Model file for the job. Use its own axes, mm. A direction names the side the tool comes from. Give positions to 0.01 mm unless a question says otherwise; leave off trailing zeros. One line per item, written item: value. Start each with the question number.
(1) Probe L1, parallel to Z at x = 12.5, y = -4.75; L2, parallel to Z at x = 19, y = -5.25; L3, parallel to X at y = -4.25, z = 24. List the from-to ranges inside material, lowest first.
(2) Cut at A-A, the plane x = -9. State how many separate pieces and enclosed holes the cut face has, and give its area (3 significant figures).
(3) 3-axis set-ups, long thin cutter, end or side, ignore diameter. For faces 4 (the face through (-29.09, -2.96, 0.19)), 5 (the face through (7, 0, -7)): which of +Z, -Z, +X, -X, +Y, -Y reach the whole face in a straight line?
(4) Mould opens along X. For faces 1 (the face through (7, -6, -7)), 2 (the face through (-6.7, -3, -0.9)), 3 (the face through (-25.07, -2.96, -19.22)) say: pulls with the +X half, pulls with the -X half, needs draft (parallel to the pull), parting line crosses it, or undercut.
from build123d import *

# Parameters (mm, degrees)
F0_R     = 31.59
F0_R_2   = 1.5
F0_R_3   = 2.5
F1_DEPTH = 6


with BuildPart() as f1:
    # F0 (on Front) → F1 (new body)
    with BuildSketch(Plane.XZ):
        Circle(F0_R)
        with BuildLine():
            ThreePointArc((5.7548407183, -28.5150821199), (-0.022576758, -29.0899912391), (-5.7990949004, -28.5061151042))
            add(Edge.make_bspline(
                [(-5.7990949004, -28.5061151042), (-3.8643270806, -24.4627677728), (0.007951806, -16.3346928963), (3.8413144045, -24.4710048156), (5.7548407183, -28.5150821199)],
                knots=[0, 0, 0, 0, 0.5002306451, 1, 1, 1, 1], degree=3))
        make_face(mode=Mode.SUBTRACT)
        with BuildLine():
            add(Edge.make_bspline(
                [(-11.5287328291, -26.7079841874), (-8.7534935922, -19.1514781576), (-3.1149871272, -3.8323867545), (-19.597387192, -6.7376991425), (-27.9114144594, -8.1964042651)],
                knots=[0, 0, 0, 0, 0.4944321997, 1, 1, 1, 1], degree=3))
            ThreePointArc((-11.5287328291, -26.7079841874), (-21.7841904219, -19.2789301483), (-27.9114144594, -8.1964042651))
        make_face(mode=Mode.SUBTRACT)
        with Locations((0, -15)):
            Circle(F0_R_2, mode=Mode.SUBTRACT)
        with Locations((0, -9)):
            Circle(F0_R_2, mode=Mode.SUBTRACT)
        with BuildLine():
            ThreePointArc((27.9114144594, -8.1964042651), (21.7841904219, -19.2789301483), (11.5287328291, -26.7079841874))
            add(Edge.make_bspline(
                [(11.5287328291, -26.7079841874), (8.7534935922, -19.1514781576), (3.1149871272, -3.8323867545), (19.597387192, -6.7376991425), (27.9114144594, -8.1964042651)],
                knots=[0, 0, 0, 0, 0.4944321997, 1, 1, 1, 1], degree=3))
        make_face(mode=Mode.SUBTRACT)
        with Locations((0, -5.5)):
            Circle(F0_R_2, mode=Mode.SUBTRACT)
        with BuildLine():
            ThreePointArc((-28.6914853437, -4.7986215489), (-29.0888528252, 0.2583434076), (-28.6017314519, 5.3074530573))
            add(Edge.make_bspline(
                [(-28.6017314519, 5.3074530573), (-24.4475826621, 4.0112175047), (-13.2248280378, -0.1559511272), (-24.4475826621, -3.6461949348), (-28.6914853437, -4.7986215489)],
                knots=[0, 0, 0, 0, 0.5017345436, 1, 1, 1, 1], degree=3))
        make_face(mode=Mode.SUBTRACT)
        with Locations((-15, 0)):
            Circle(F0_R_2, mode=Mode.SUBTRACT)
        with Locations((-9, 0)):
            Circle(F0_R_2, mode=Mode.SUBTRACT)
        with Locations((-5.5, 0)):
            Circle(F0_R_2, mode=Mode.SUBTRACT)
        with BuildLine():
            ThreePointArc((-27.9114144594, 8.1964042651), (-21.7841904219, 19.2789301483), (-11.5287328291, 26.7079841874))
            add(Edge.make_bspline(
                [(-11.5287328291, 26.7079841874), (-8.7534935922, 19.1514781576), (-3.1149871272, 3.8323867545), (-19.597387192, 6.7376991425), (-27.9114144594, 8.1964042651)],
                knots=[0, 0, 0, 0, 0.4944321997, 1, 1, 1, 1], degree=3))
        make_face(mode=Mode.SUBTRACT)
        with BuildLine():
            add(Edge.make_bspline(
                [(-5.7990949004, 28.5061151042), (-3.8643270806, 24.4627677728), (0.007951806, 16.3346928963), (3.8413144045, 24.4710048156), (5.7548407183, 28.5150821199)],
                knots=[0, 0, 0, 0, 0.5002306451, 1, 1, 1, 1], degree=3))
            ThreePointArc((-5.7990949004, 28.5061151042), (-0.022576758, 29.0899912391), (5.7548407183, 28.5150821199))
        make_face(mode=Mode.SUBTRACT)
        Circle(F0_R_3, mode=Mode.SUBTRACT)
        with Locations((5.5, 0)):
            Circle(F0_R_2, mode=Mode.SUBTRACT)
        with Locations((0, 5.5)):
            Circle(F0_R_2, mode=Mode.SUBTRACT)
        with Locations((9, 0)):
            Circle(F0_R_2, mode=Mode.SUBTRACT)
        with Locations((15, 0)):
            Circle(F0_R_2, mode=Mode.SUBTRACT)
        with Locations((0, 9)):
            Circle(F0_R_2, mode=Mode.SUBTRACT)
        with Locations((0, 15)):
            Circle(F0_R_2, mode=Mode.SUBTRACT)
        with BuildLine():
            add(Edge.make_bspline(
                [(11.5287328291, 26.7079841874), (8.7534935922, 19.1514781576), (3.1149871272, 3.8323867545), (19.597387192, 6.7376991425), (27.9114144594, 8.1964042651)],
                knots=[0, 0, 0, 0, 0.4944321997, 1, 1, 1, 1], degree=3))
            ThreePointArc((11.5287328291, 26.7079841874), (21.7841904219, 19.2789301483), (27.9114144594, 8.1964042651))
        make_face(mode=Mode.SUBTRACT)
        with BuildLine():
            add(Edge.make_bspline(
                [(28.6017314519, 5.3074530573), (24.4475826621, 4.0112175047), (13.2248280378, -0.1559511272), (24.4475826621, -3.6461949348), (28.6914853437, -4.7986215489)],
                knots=[0, 0, 0, 0, 0.5017345436, 1, 1, 1, 1], degree=3))
            ThreePointArc((28.6017314519, 5.3074530573), (29.0888528252, 0.2583434076), (28.6914853437, -4.7986215489))
        make_face(mode=Mode.SUBTRACT)
    extrude(amount=F1_DEPTH)


solid = f1.part
Answers follow:
1. L1: z = -29.01 to -26.27, -6.7 to 6.7, 26.27 to 29.01
1. L2: z = -25.24 to -22.03, -6.81 to -0.56, 0.59 to 6.81, 22.03 to 25.24
1. L3: x = -20.54 to -16.44, -10.54 to -3.53, 3.51 to 10.54, 16.44 to 20.54
2. separate pieces: 4
2. enclosed holes: 0
2. area: 208 mm²
3. face 4: +Y, -Y
3. face 5: +Z, -Z, +X, -X, +Y
4. face 1: needs draft
4. face 2: undercut
4. face 3: parting line crosses it
